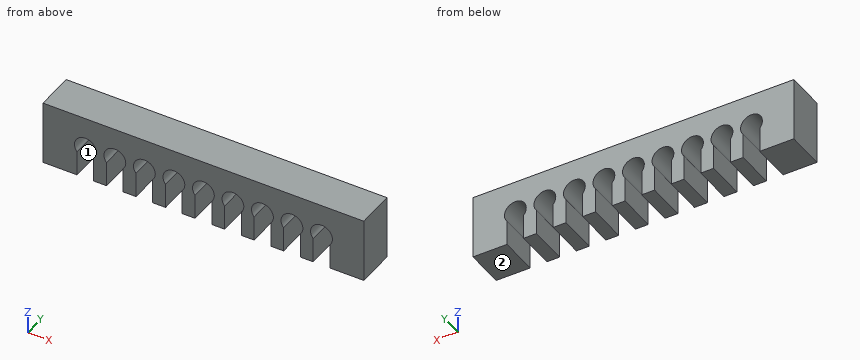
from build123d import *

# Parameters (mm, degrees)
CROQUIS1_W              = 25
CROQUIS1_H              = 5
SALIENTE_EXTRUIR1_DEPTH = 3
CORTAR_EXTRUIR6_DEPTH   = 3
MATRIZL4_COUNT          = 5
MATRIZL4_PITCH          = 2.3
SIMETR_A3_COPY_1_DEPTH  = 3
SIMETR_A3_COPY_2_DEPTH  = 3
SIMETR_A3_COPY_3_DEPTH  = 3
SIMETR_A3_COPY_4_DEPTH  = 3
SIMETR_A3_COPY_5_DEPTH  = 3


with BuildPart() as part:
    # Croquis1 → Saliente-Extruir1 (new body)
    with BuildSketch(Plane(origin=(0, 0, 0), x_dir=(1, 0, 0), z_dir=(0, 1, 0))):
        Rectangle(CROQUIS1_W, CROQUIS1_H)
    extrude(amount=SALIENTE_EXTRUIR1_DEPTH)

    # Croquis2 → Cortar-Extruir6 (cut)
    with BuildSketch(Plane(origin=(0, 3, 0), x_dir=(1, 0, 0), z_dir=(0, 1, 0))):
        with BuildLine():
            Line((0.65, 0.547722558), (0.65, 2.5))
            Line((0.65, 2.5), (-0.65, 2.5))
            Line((-0.65, 2.5), (-0.65, 0.547722558))
            ThreePointArc((-0.65, 0.547722558), (0, -0.85), (0.65, 0.547722558))
        make_face()
    cortar_extruir6 = extrude(amount=-CORTAR_EXTRUIR6_DEPTH, mode=Mode.SUBTRACT)

    # MatrizL4: Cortar-Extruir6 ×5
    with Locations(*[(i * MATRIZL4_PITCH, 0, 0) for i in range(1, MATRIZL4_COUNT)]):
        add(cortar_extruir6, mode=Mode.SUBTRACT)

    # Simetría3 copy 1 sketch → Simetría3 copy 1 (cut)
    with BuildSketch(Plane(origin=(-2.3, 3, 0), x_dir=(-1, 0, 0), z_dir=(0, 1, 0))):
        with BuildLine():
            Line((0.65, -0.547722558), (0.65, -2.5))
            Line((0.65, -2.5), (-0.65, -2.5))
            Line((-0.65, -2.5), (-0.65, -0.547722558))
            ThreePointArc((-0.65, -0.547722558), (0, 0.85), (0.65, -0.547722558))
        make_face()
    extrude(amount=-SIMETR_A3_COPY_1_DEPTH, mode=Mode.SUBTRACT)

    # Simetría3 copy 2 sketch → Simetría3 copy 2 (cut)
    with BuildSketch(Plane(origin=(-4.6, 3, 0), x_dir=(-1, 0, 0), z_dir=(0, 1, 0))):
        with BuildLine():
            Line((0.65, -0.547722558), (0.65, -2.5))
            Line((0.65, -2.5), (-0.65, -2.5))
            Line((-0.65, -2.5), (-0.65, -0.547722558))
            ThreePointArc((-0.65, -0.547722558), (0, 0.85), (0.65, -0.547722558))
        make_face()
    extrude(amount=-SIMETR_A3_COPY_2_DEPTH, mode=Mode.SUBTRACT)

    # Simetría3 copy 3 sketch → Simetría3 copy 3 (cut)
    with BuildSketch(Plane(origin=(-6.9, 3, 0), x_dir=(-1, 0, 0), z_dir=(0, 1, 0))):
        with BuildLine():
            Line((0.65, -0.547722558), (0.65, -2.5))
            Line((0.65, -2.5), (-0.65, -2.5))
            Line((-0.65, -2.5), (-0.65, -0.547722558))
            ThreePointArc((-0.65, -0.547722558), (0, 0.85), (0.65, -0.547722558))
        make_face()
    extrude(amount=-SIMETR_A3_COPY_3_DEPTH, mode=Mode.SUBTRACT)

    # Simetría3 copy 4 sketch → Simetría3 copy 4 (cut)
    with BuildSketch(Plane(origin=(-9.2, 3, 0), x_dir=(-1, 0, 0), z_dir=(0, 1, 0))):
        with BuildLine():
            Line((0.65, -0.547722558), (0.65, -2.5))
            Line((0.65, -2.5), (-0.65, -2.5))
            Line((-0.65, -2.5), (-0.65, -0.547722558))
            ThreePointArc((-0.65, -0.547722558), (0, 0.85), (0.65, -0.547722558))
        make_face()
    extrude(amount=-SIMETR_A3_COPY_4_DEPTH, mode=Mode.SUBTRACT)

    # Simetría3 copy 5 sketch → Simetría3 copy 5 (cut)
    with BuildSketch(Plane(origin=(0, 3, 0), x_dir=(-1, 0, 0), z_dir=(0, 1, 0))):
        with BuildLine():
            Line((0.65, -0.547722558), (0.65, -2.5))
            Line((0.65, -2.5), (-0.65, -2.5))
            Line((-0.65, -2.5), (-0.65, -0.547722558))
            ThreePointArc((-0.65, -0.547722558), (0, 0.85), (0.65, -0.547722558))
        make_face()
    extrude(amount=-SIMETR_A3_COPY_5_DEPTH, mode=Mode.SUBTRACT)


solid = part.part
Can you work these out from the model? Positions are in its coordinate system, mm. Face numbers are marked on the shaded views. A direction names the side the tool comes from. Round coordinates to 2 decimals unless told otherwise and drop trailing zeros. Order: outer loops, then holes, each group sorted by start corner. A loop starts at its lowest first (then second) coordinate and runs counter-clockwise, first axis right, second up. Notation, with made-up numbers: (20.5, 68.25) -> (49.5, 68.25) arc R18 ccw to (49.5, 73.25) -> close; hole circle Ø11 at (8.25, 29.25). An arc over 180 degrees is marked (long way). Write each question's results on one line, items separated by ' | '. Start each with the question number.
Item 1: Please list where these lines run through material, in increasing order: L1, parallel to Z at x = -9.2, y = 1.25; L2, parallel to Z at x = 8.5, y = 1.85.
Item 2: If we section it at A-A, the plane z = 0: State how many separate pieces and enclosed holes the cut face has, then the cut area to 3 significant figures.
Item 3: Which directions (+Z, -Z, +X, -X, +Y, -Y) give clear straight access to the entire face, cutting with the end or side of a thin tool? Please do the marked faces 1 and 2.
Item 4: If we section it at D-D, the plane x = -9.2: Write out the boundary of the cut face in (y, z), then the cut area to 3 significant figures.
Item 5: If we section it at B-B, the plane x = -5: Write out the boundary of the cut face in (y, z).
Results:
1) L1: z = 0.85 to 2.5 | L2: z = -2.5 to -0.48, 0.48 to 2.5
2) separate pieces: 10 | enclosed holes: 0 | area: 29.1 mm2
3) face 1: -Z, +Y, -Y | face 2: -Z, +X, -X, +Y, -Y
4) outline: (0, 0.85) -> (3, 0.85) -> (3, 2.5) -> (0, 2.5) -> close | area: 4.95 mm2
5) outline: (0, 0.75) -> (3, 0.75) -> (3, 2.5) -> (0, 2.5) -> close
